Job drawing, mm, ordinate dimensions from the low corner. One solid piece. Coordinates: 2 decimals unless noted, no trailing zeros. Loops run counter-clockwise (first coordinate to the right, second up) from the corner with the lowest first, then second, coordinate; pieces in that order, holes last. Notation, with made-up numbers: (46.25, -26) - (57.25, -26) arc R23 ccw to (57.25, -15) - close; hole circle Ø2 at (62, -35.5). An arc over 180 degrees is marked (long way). Use a Markdown table: item, result. Add a question column.
1) Band-saw the part on D-D (y = 11.29). Give the cut face in (x, z).
2) Band-saw the part on B-B (y = 26). Give the cut face in (x, z).
3) Band-saw the part on A-A (z = 31.5). Give the cut face in (x, y), plus the area to 3 significant figures.
4) Drop flat-ended pins along their axis: P1, Ø4, axis at y = 11.29, z = 2.54, coming from the +X side; P2, Ø6, axis at y = 12, z = 62.5, coming from the +X side; P3, Ø2, axis at x = 1.5, y = 5, coming from the -Z side; P4, Ø1.3, axis at x = 1, z = 19, coming from the -Y side. Give the stop position or say it passes through.
5) Band-saw the part on C-C (x = 0.95). Give the cut face in (y, z), plus the area to 4 significant figures.
6) Probe probe 1 along Z at (x, y) = (0.95, 11.29); probe 2 along Z at (x, y) = (3.35, 22.5); probe 3 along Y at (x, z) = (3.05, 60.5). List the from-to ranges inside material, lowest first. Write a range as [from, to].
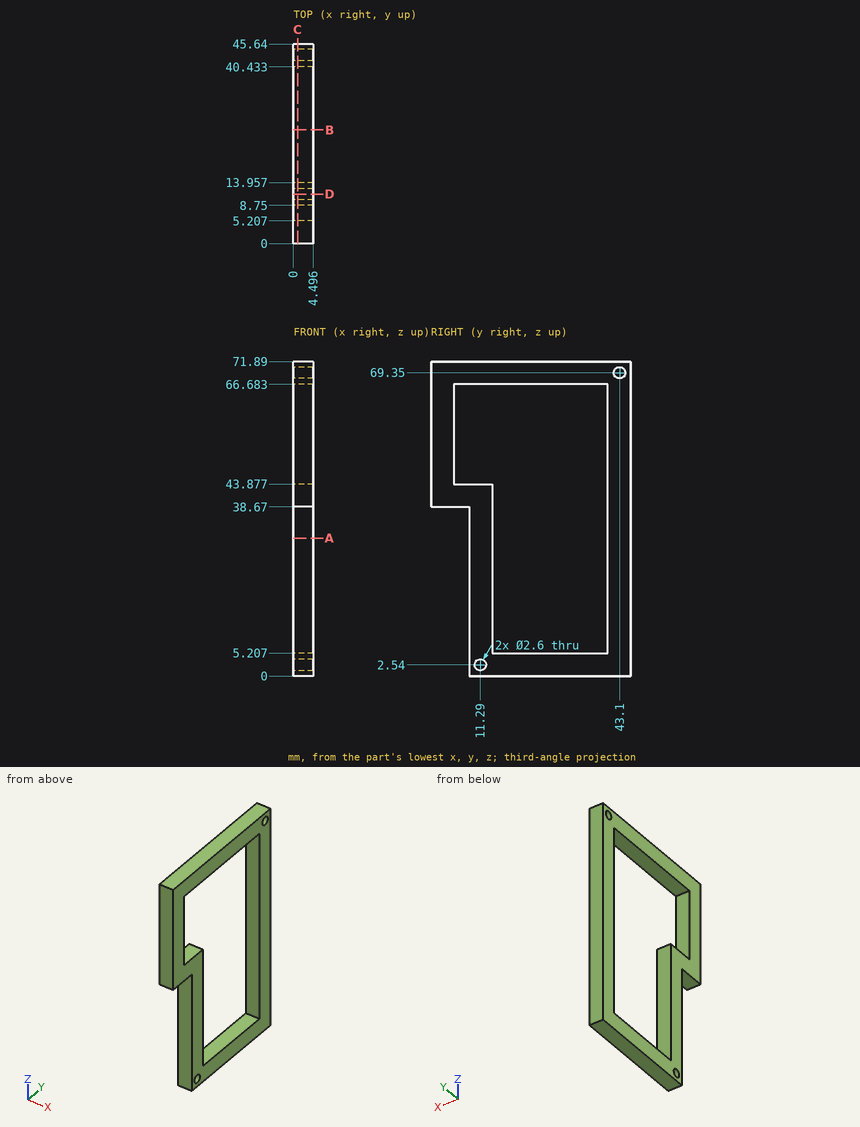
Answer block:
| question | item | result |
|---|---|---|
| 1 | outline | (0, 0) - (4.5, 0) - (4.5, 1.24) - (0, 1.24) - close; (0, 3.84) - (4.5, 3.84) - (4.5, 43.88) - (0, 43.88) - close; (0, 66.68) - (4.5, 66.68) - (4.5, 71.89) - (0, 71.89) - close |
| 2 | outline | (0, 0) - (4.5, 0) - (4.5, 5.21) - (0, 5.21) - close; (0, 66.68) - (4.5, 66.68) - (4.5, 71.89) - (0, 71.89) - close |
| 3 | outline | (0, 8.75) - (4.5, 8.75) - (4.5, 13.96) - (0, 13.96) - close; (0, 40.43) - (4.5, 40.43) - (4.5, 45.64) - (0, 45.64) - close |
| 3 | area | 46.8 mm2 |
| 4 | P1 | x = 4.5 |
| 4 | P2 | through |
| 4 | P3 | z = 38.67 |
| 4 | P4 | y = 8.75 |
| 5 | outline | (0, 38.67) - (8.75, 38.67) - (8.75, 0) - (45.64, 0) - (45.64, 71.89) - (0, 71.89) - close; hole (5.21, 43.88) - (13.96, 43.88) - (13.96, 5.21) - (40.43, 5.21) - (40.43, 66.68) - (5.21, 66.68) - close; hole circle Ø2.6 at (11.29, 2.54); hole circle Ø2.6 at (43.1, 69.35) |
| 5 | area | 1,105 mm2 |
| 6 | probe 1 | [0, 1.24], [3.84, 43.88], [66.68, 71.89] |
| 6 | probe 2 | [0, 5.21], [66.68, 71.89] |
| 6 | probe 3 | [0, 5.21], [40.43, 45.64] |
